Geometry: final body of the model. Coordinates: model frame, mm. Give positions to 0.01 mm unless a question says otherwise; leave off trailing zeros. Use CSV: the item, a comma, the result in double quotes. Start each with the question number.
1) Material intervals for line 1 (Y direction, x = -24, z = 2.9); line 2 (X direction, y = -42.5, z = 2.1); line 3 (X direction, y = 41, z = 1.75), sorted ascending. Write a range as [from, to].
2) Contact query for flat-ended pins moving along their axis: P1, Ø2, axis at y = 46.5, z = 3.5, coming from the -X side; P2, Ø1.5, axis at x = 11, z = 3.5, coming from the +Y side; P3, Ø1.2, axis at y = -46.5, z = 2.5, coming from the +X side; P4, Ø2.5, axis at x = 25, y = 41.5, coming from the +Z side. Output: stop coordinate, or through.
3) Section A-A (z = 1.4). Count the separate pieces of the cut face and the enclosed holes in it, plus the area to 3 significant figures.
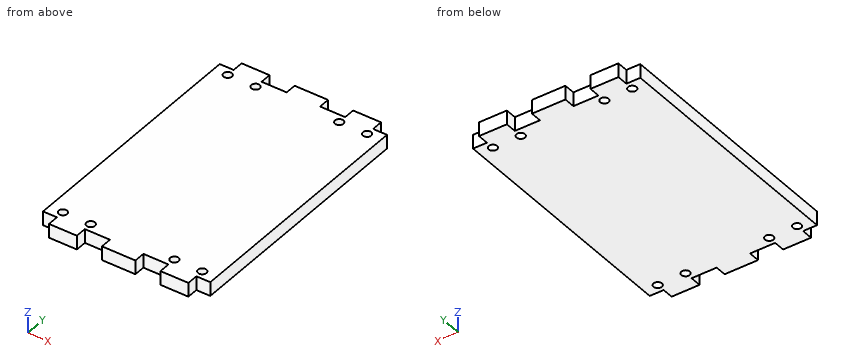
```python
from build123d import *

# Parameters (mm, degrees)
SKETCH_1_W          = 60
SKETCH_1_H          = 97
EXTRUDE_1_DEPTH     = 5
SKETCH_2_OUTSIDE_W  = 84.834
SKETCH_2_OUTSIDE_H  = 121.834
CUT_EXTRUDE_1_DEPTH = 10
SKETCH_3_R          = 1.5
CUT_EXTRUDE_2_DEPTH = 10


with BuildPart() as part:
    # 草图1 → 凸台-拉伸1 (new body)
    with BuildSketch(Plane.XY):
        Rectangle(SKETCH_1_W, SKETCH_1_H)
    extrude(amount=EXTRUDE_1_DEPTH)

    # 草图2 outside → 切除-拉伸1 (cut)
    with BuildSketch(Plane.XY.offset(5)):
        Rectangle(SKETCH_2_OUTSIDE_W, SKETCH_2_OUTSIDE_H)
        Polygon((6, 48.5), (-6, 48.5), (-6, 44.5), (-15, 44.5), (-15, 48.5), (-25, 48.5), (-25, 44.5), (-30, 44.5), (-30, -44.5), (-25, -44.5), (-25, -48.5), (-15, -48.5), (-15, -44.5), (-6, -44.5), (-6, -48.5), (6, -48.5), (6, -44.5), (15, -44.5), (15, -48.5), (25, -48.5), (25, -44.5), (30, -44.5), (30, 44.5), (25, 44.5), (25, 48.5), (15, 48.5), (15, 44.5), (6, 44.5), align=None, mode=Mode.SUBTRACT)
    extrude(amount=-CUT_EXTRUDE_1_DEPTH, mode=Mode.SUBTRACT)

    # 草图3 → 切除-拉伸2 (cut)
    with BuildSketch(Plane.XY.offset(5)):
        with Locations((-25, 41.5)):
            Circle(SKETCH_3_R)
        with Locations((-15.000001244, 41.504987561)):
            Circle(SKETCH_3_R)
        with Locations((15.000001244, 41.504987561)):
            Circle(SKETCH_3_R)
        with Locations((25, 41.5)):
            Circle(SKETCH_3_R)
        with Locations((25, -41.5)):
            Circle(SKETCH_3_R)
        with Locations((15.000001244, -41.504987561)):
            Circle(SKETCH_3_R)
        with Locations((-15.000001244, -41.504987561)):
            Circle(SKETCH_3_R)
        with Locations((-25, -41.5)):
            Circle(SKETCH_3_R)
    extrude(amount=-CUT_EXTRUDE_2_DEPTH, mode=Mode.SUBTRACT)


solid = part.part
```
Answers follow:
1,line 1,"y = [-48.5, -42.62], [-40.38, 40.38], [42.62, 48.5]"
1,line 2,"x = [-30, -26.12], [-23.88, -16.12], [-13.88, 13.88], [16.12, 23.88], [26.12, 30]"
1,line 3,"x = [-30, -26.41], [-23.59, -16.41], [-13.59, 13.59], [16.41, 23.59], [26.41, 30]"
2,P1,"stops at x = -25"
2,P2,"stops at y = 44.5"
2,P3,"stops at x = 25"
2,P4,"passes through"
3,separate pieces,"1"
3,enclosed holes,"8"
3,area,"5,540 mm^2"
